Geometry: final body of the model. Coordinates: model frame, mm. Give positions to 0.01 mm unless a question says otherwise; leave off trailing zeros. Loops run counter-clockwise (first coordinate to the right, second up) from the corner with the lowest first, then second, coordinate; pieces in that order, holes last. Notation, with made-up numbers: (-13, 11) -> (43, 11) arc R34 cw to (43, 41) -> close; hole circle Ø11 at (-31.75, 73.25). An arc over 180 degrees is marked (long way). Answer in a Markdown table with one row per item. Add a question column.
1) First-contact query: P1, Ø1, axis at x = 43, y = 1.5, coming from the +Z side; P2, Ø1, axis at y = 2, z = -54.5, coming from the +X side (3 decimals); P3, Ø1.6, axis at y = 2, z = -5.5, coming from the -X side. Flat tips, straight axial feed; report the tip coordinate or a pass-through.
2) Section query D-D (z = -33.5). Return the cut outline in (x, y) (3 decimals), plus the area to 3 significant figures.
3) Line query: line 1 (X direction, y = 0.85, z = -29); line 2 (X direction, y = 2, z = -19.05) (3 decimals); line 3 (Z direction, x = 42, y = 1.8). Output: solid intervals per line, ascending. Write a range as from..to.
4) Section query C-C (x = 11). Return the cut outline in (y, z) (3 decimals).
5) Section query A-A (z = -19.05). Return the cut outline in (x, y) (3 decimals).
6) Section query B-B (y = 1.3). Give the number of separate pieces and of enclosed holes in the cut face, plus the area to 3 significant figures.
```python
from build123d import *

# Parameters (mm, degrees)
SKETCH1_W            = 3.175
SKETCH1_H            = 7.62
BOSS_EXTRUDE1_DEPTH  = 3.175
M3_CLEARANCE_HOLE1_D = 3.2


with BuildPart() as part:
    # Sketch1 → Boss-Extrude1 (new body)
    with BuildSketch(Plane(origin=(0, 0, 0), x_dir=(1, 0, 0), z_dir=(0, 1, 0))):
        Polygon((0, 0), (13.335, 0), (13.335, -3.175), (32.385, -3.175), (32.385, 0), (45.72, 0), (45.72, 52.78882), (32.385, 52.78882), (32.385, 55.96382), (13.335, 55.96382), (13.335, 52.78882), (0, 52.78882), (0, 28.575), (-3.175, 28.575), (-3.175, 9.525), (0, 9.525), align=None)
        with Locations((42.545, 26.67)):
            Rectangle(SKETCH1_W, SKETCH1_H, mode=Mode.SUBTRACT)
        with Locations((42.545, 11.43)):
            Rectangle(SKETCH1_W, SKETCH1_H, mode=Mode.SUBTRACT)
    extrude(amount=BOSS_EXTRUDE1_DEPTH)

    # M3 Clearance Hole1 (through all)
    with Locations(Plane(origin=(0, 3.175, 0), x_dir=(1, 0, 0), z_dir=(0, 1, 0))):
        with Locations((42.545, 19.05)):
            Hole(M3_CLEARANCE_HOLE1_D / 2)


solid = part.part
```
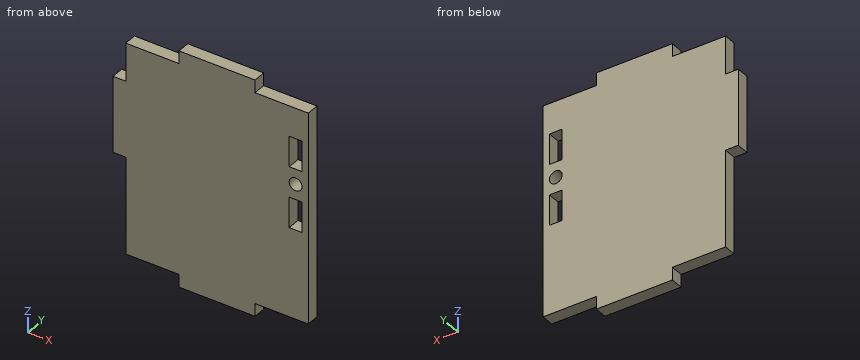
Evaluation:
| question | item | result |
|---|---|---|
| 1 | P1 | z = 0 |
| 1 | P2 | x = 32.385 |
| 1 | P3 | x = 0 |
| 2 | outline | (0, 0) -> (45.72, 0) -> (45.72, 3.175) -> (0, 3.175) -> close |
| 2 | area | 145 mm² |
| 3 | line 1 | 0..40.96, 44.13..45.72 |
| 3 | line 2 | -3.175..40.945, 44.145..45.72 |
| 3 | line 3 | -52.79..-30.48, -22.86..-20.55, -17.55..-15.24, -7.62..0 |
| 4 | outline | (0, -52.789) -> (3.175, -52.789) -> (3.175, 0) -> (0, 0) -> close |
| 5 | outline | (-3.175, 0) -> (40.945, 0) -> (40.945, 3.175) -> (-3.175, 3.175) -> close; (44.145, 0) -> (45.72, 0) -> (45.72, 3.175) -> (44.145, 3.175) -> close |
| 6 | separate pieces | 1 |
| 6 | enclosed holes | 3 |
| 6 | area | 2,540 mm² |
